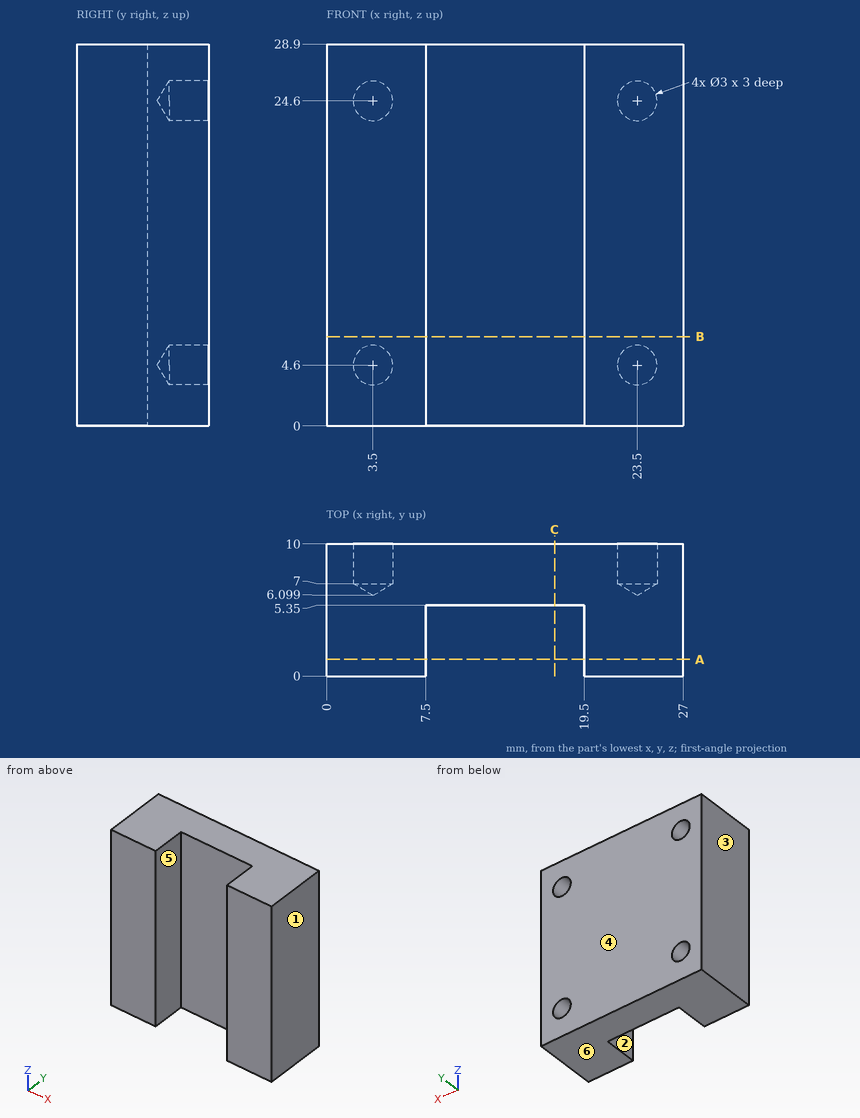
The figure shows three views and two pictorial views of one solid part (mm, origin at its lowest corner). Answer the questions. A direction names the side the tool comes from. Round coordinates to 2 decimals unless told otherwise and drop trailing zeros. Loops run counter-clockwise (first coordinate to the right, second up) from the corner with the lowest first, then second, coordinate; pieces in that order, holes last. Notation, with made-up numbers: (56.25, 38) -> (73.25, 38) arc R18 ccw to (73.25, 69) -> close; hole circle Ø2 at (69, -35). An arc over 180 degrees is marked (long way). Use one line per item in the form item = value.
(1) A tool of negligible diameter and unlimited length cuts with its end or side. For the marked faces 5 and 6, from which of +Z, -Z, +X, -X, +Y, -Y can it reach the whole face along a straight path? Write none if from no direction.
Answer list:
face_5 = +Z, -Z, -Y
face_6 = -Z, +X, -X, +Y, -Y
(2) Straight lines are drawn through the part: line 1 (Z direction, x = 3.5, y = 9.25); line 2 (X direction, y = 9.1, z = 24.6); line 3 (X direction, y = 2.25, z = 6). For each, find the intervals that lie inside material, in ascending order.
Answer list:
line_1 = 0 to 3.1, 6.1 to 23.1, 26.1 to 28.9
line_2 = 0 to 2, 5 to 22, 25 to 27
line_3 = 0 to 7.5, 19.5 to 27
(3) Find section A-A on y = 1.25. Give the vertices of the cut face in (x, z).
Answer list:
outline = (0, 0) -> (7.5, 0) -> (7.5, 28.9) -> (0, 28.9) -> close; (19.5, 0) -> (27, 0) -> (27, 28.9) -> (19.5, 28.9) -> close
(4) For a pull along X with two mould halves and no side action, classify the marked faces 1, 2, 3 and 4 as released by +X, released by -X, zero draft, split by the parting line, or undercut.
Answer list:
face_1 = released by +X
face_2 = undercut
face_3 = released by -X
face_4 = zero draft
(5) Find section B-B on z = 6.75. Give the vertices of the cut face in (x, y).
Answer list:
outline = (0, 0) -> (7.5, 0) -> (7.5, 5.35) -> (19.5, 5.35) -> (19.5, 0) -> (27, 0) -> (27, 10) -> (0, 10) -> close
(6) Find section C-C on x = 17.25. Give the vertices of the cut face in (y, z), then the cut area to 3 significant figures.
Answer list:
outline = (5.35, 0) -> (10, 0) -> (10, 28.9) -> (5.35, 28.9) -> close
area = 134 mm2
(7) Flat-ended cylindrical pins translate along their axes: P1, Ø5, axis at x = 3.5, z = 4.6, coming from the -Y side; P2, Ø5, axis at x = 10.5, z = 8.5, coming from the -Y side. Find the tip coordinate at first contact, or state that the pin passes through.
Answer list:
P1 = 0
P2 = 5.35
